from build123d import *


with BuildPart() as part:
    # Croquis1 → Revolución1 (revolve)
    with BuildSketch(Plane.XY, mode=Mode.PRIVATE) as revoluci_n1_sk:
        Polygon((0, 68.35), (26.6, 68.35), (26.6, 56.15), (15.85, 56.15), (15.85, -53.85), (14.35, -55.35), (14.35, -57.35), (15.85, -58.85), (15.85, -64.45), (15, -68.35), (0, -68.35), align=None)
    revolve(revoluci_n1_sk.sketch.rotate(Axis((0, 107.931381584, 0), (0, -1, 0)), 90), axis=Axis((0, 107.931381584, 0), (0, -1, 0)))


solid = part.part
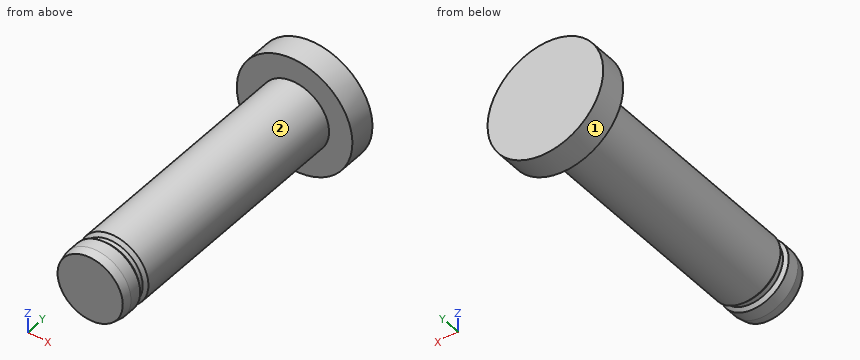
Geometry check sheet. Reference: the model listing, model coordinates, mm. Face numbers are marked on the shaded views. A direction names the side the tool comes from. Round coordinates to 2 decimals unless told otherwise and drop trailing zeros. Write each loop counter-clockwise with the first axis right and the second up, starting at its lowest first coordinate (ties: lowest second). Pieces come first, ordered by that corner, then holes.
Item 1: Access from +Z, -Z, +X, -X, +Y, -Y to the whole of each face (thin tool, end or side, straight path). Record for the marked faces 1 and 2.
Determined:
face 1: +Y, -Y
face 2: -Y
Item 2: Section check A-A (z = 0). Record the boundary of the cut face in (x, y).
Determined:
outline: (-26.6, 56.15) - (-15.85, 56.15) - (-15.85, -53.85) - (-14.35, -55.35) - (-14.35, -57.35) - (-15.85, -58.85) - (-15.85, -64.45) - (-15, -68.35) - (15, -68.35) - (15.85, -64.45) - (15.85, -58.85) - (14.35, -57.35) - (14.35, -55.35) - (15.85, -53.85) - (15.85, 56.15) - (26.6, 56.15) - (26.6, 68.35) - (-26.6, 68.35) - close
Item 3: Section check B-B (x = 0). Record the boundary of the cut face in (y, z), plus the area to 3 significant figures.
Determined:
outline: (-68.35, -15) - (-64.45, -15.85) - (-58.85, -15.85) - (-57.35, -14.35) - (-55.35, -14.35) - (-53.85, -15.85) - (56.15, -15.85) - (56.15, -26.6) - (68.35, -26.6) - (68.35, 26.6) - (56.15, 26.6) - (56.15, 15.85) - (-53.85, 15.85) - (-55.35, 14.35) - (-57.35, 14.35) - (-58.85, 15.85) - (-64.45, 15.85) - (-68.35, 15) - close
area: 4,580 mm2
Item 4: Material ranges on line 1 along Y through (x, z) = (17.5, 11.5); line 2 along Z through (x, y) = (-2, 9); line 3 along X through (y, z) = (20, -6), recorded low to high.
Determined:
line 1: y = 56.15 to 68.35
line 2: z = -15.72 to 15.72
line 3: x = -14.67 to 14.67
Item 5: Go/stop test with flat-tipped pins: pin 1 Ø8 at (x, y) = (0, 40) entering from -Z; pin 2 Ø2 at (y, z) = (0.5, 1) entering from -X; pin 3 Ø8 at (x, y) = (-1.5, 47) entering from +Z; pin 4 Ø2 at (y, z) = (-47.5, 18) entering from -X. Record where each tip stops, or that it passes through.
Determined:
pin 1: stops at z = -15.85
pin 2: stops at x = -15.85
pin 3: stops at z = 15.85
pin 4: passes through
Item 6: Section check D-D (z = 17.5). Record the boundary of the cut face in (x, y).
Determined:
outline: (-20.03, 56.15) - (20.03, 56.15) - (20.03, 68.35) - (-20.03, 68.35) - close
Item 7: Section check C-C (y = 10.5). Record the boundary of the cut face in (x, z).
Determined:
outline: circle Ø31.7 at (0, 0)
